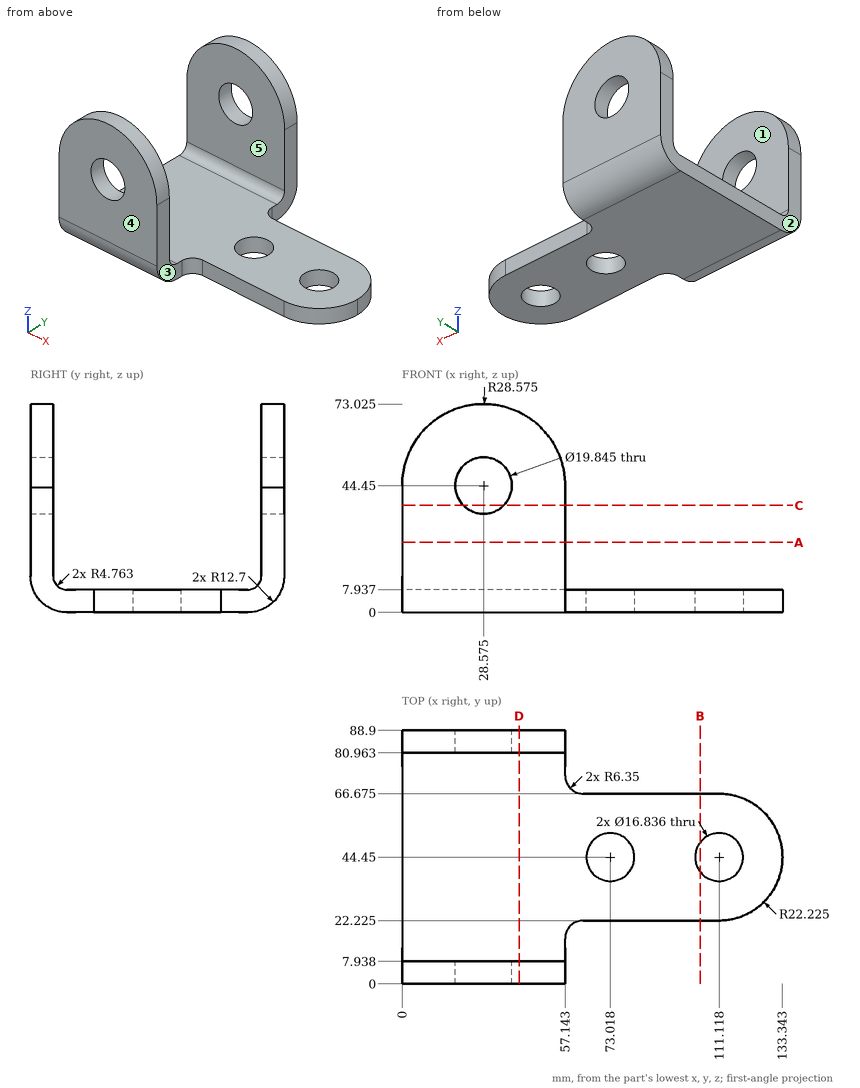
Drawing for the job (mm, zero at the part's lowest x, y, z). A direction names the side the tool comes from. Coordinates: 2 decimals unless noted, no trailing zeros. Loops run counter-clockwise (first coordinate to the right, second up) from the corner with the lowest first, then second, coordinate; pieces in that order, holes last. Notation, with made-up numbers: (8, -33.5) - (38, -33.5) arc R27 cw to (38, -6.5) - close; hole circle Ø7 at (10, 42.25). An arc over 180 degrees is marked (long way). Return JSON: item names as keys, results as strings.
1. Probe L1, parallel to X at y = 44, z = 6 (1 decimal); L2, parallel to Y at x = 16, z = 14.5; L3, parallel to Z at x = 43, y = 17.5. List the from-to ranges inside material, lowest first. Write a range as from..to.
Result:
{"L1": "x = 0..64.6, 81.4..102.7, 119.5..133.3", "L2": "y = 0..7.94, 80.96..88.9", "L3": "z = 0..7.94"}
2. Drop flat-ended pins along their axis: pin 1 (8 mm diameter, centred on x = 116, y = 47, fed in from -Z); pin 2 (4 mm diameter, centred on x = 76.5, z = 4, fed in from -Y) (1 decimal); pin 3 (13.5 mm diameter, centred on x = 111.12, y = 44.45, fed in from -Z); pin 4 (6.5 mm diameter, centred on x = 77.5, z = 6, fed in from +Y) (1 decimal). Give the stop position or say it passes through.
Result:
{"pin 1": "stops at z = 0", "pin 2": "stops at y = 22.2", "pin 3": "passes through", "pin 4": "stops at y = 66.7"}
3. Band-saw the part on B-B (x = 104.5). Give the cut face in (y, z) (1 decimal).
Result:
{"outline": "(22.2, 0) - (39.2, 0) - (39.2, 7.9) - (22.2, 7.9) - close; (49.7, 0) - (66.7, 0) - (66.7, 7.9) - (49.7, 7.9) - close"}
4. Band-saw the part on A-A (z = 24.5). Give the cut face in (x, y).
Result:
{"outline": "(0, 0) - (57.14, 0) - (57.14, 7.94) - (0, 7.94) - close; (0, 80.96) - (57.14, 80.96) - (57.14, 88.9) - (0, 88.9) - close"}
5. Mould opens along Y. For the marked faces 3, 4 and 5 say: released by +Y, released by -Y, zero draft, split by the parting line, or undercut.
Result:
{"face 3": "zero draft", "face 4": "released by -Y", "face 5": "undercut"}
6. 3-axis set-ups, long thin cutter, end or side, ignore diameter. For the marked faces 1 and 2: which of +Z, -Z, +X, -X, +Y, -Y reach the whole face in a straight line?
Result:
{"face 1": "+Z, +X, -X", "face 2": "+Z, -Z, -X, +Y, -Y"}
7. Band-saw the part on C-C (z = 37.5). Give the cut face in (x, y).
Result:
{"outline": "(0, 0) - (21.49, 0) - (21.49, 7.94) - (0, 7.94) - close; (0, 80.96) - (21.49, 80.96) - (21.49, 88.9) - (0, 88.9) - close; (35.66, 0) - (57.14, 0) - (57.14, 7.94) - (35.66, 7.94) - close; (35.66, 80.96) - (57.14, 80.96) - (57.14, 88.9) - (35.66, 88.9) - close"}
8. Band-saw the part on D-D (x = 41). Give the cut face in (y, z) (1 decimal), and give its area (3 significant figures).
Result:
{"outline": "(0, 12.7) arc R12.7 ccw to (12.7, 0) - (76.2, 0) arc R12.7 ccw to (88.9, 12.7) - (88.9, 70.2) - (81, 70.2) - (81, 12.7) arc R4.8 cw to (76.2, 7.9) - (12.7, 7.9) arc R4.8 cw to (7.9, 12.7) - (7.9, 70.2) - (0, 70.2) - close", "area": "1,630 mm2"}
